from build123d import *

# Parameters (mm, degrees)
MAIN_LID_SKETCH_W   = 76.2
MAIN_LID_SKETCH_H   = 53.975
MAIN_LID_DEPTH      = 2.54
HOLE_CUT_DEPTH      = 47.758814744
HOLE_CUT_DEPTH_BACK = 47.758814744
HOLE_CUT_SKETCH_R   = 3.175
CORNER_FILLET_R     = 6.35


with BuildPart() as part:
    # Main Lid Sketch → Main Lid (new body)
    with BuildSketch(Plane(origin=(0, 0, 0), x_dir=(1, 0, 0), z_dir=(0, 1, 0))):
        Rectangle(MAIN_LID_SKETCH_W, MAIN_LID_SKETCH_H)
    extrude(amount=MAIN_LID_DEPTH)

    # Hole Cut Sketch → Hole Cut (cut, two sides: drawn at the far end of the back side and taken through both)
    with BuildSketch(Plane(origin=(0, 2.54, 0), x_dir=(1, 0, 0), z_dir=(0, 1, 0)).offset(-HOLE_CUT_DEPTH_BACK)):
        with Locations(Location((31.75, -20.6375, 0), (0, 0, 270))):
            Circle(HOLE_CUT_SKETCH_R)
        with Locations(Location((22.225, -20.6375, 0), (0, 0, 270))):
            Circle(HOLE_CUT_SKETCH_R)
        with Locations(Location((-31.75, -20.6375, 0), (0, 0, 270))):
            Circle(HOLE_CUT_SKETCH_R)
        with Locations(Location((-31.75, 20.6375, 0), (0, 0, 270))):
            Circle(HOLE_CUT_SKETCH_R)
        with Locations(Location((22.225, 20.6375, 0), (0, 0, 270))):
            Circle(HOLE_CUT_SKETCH_R)
        with Locations(Location((31.75, 20.6375, 0), (0, 0, 270))):
            Circle(HOLE_CUT_SKETCH_R)
    extrude(amount=HOLE_CUT_DEPTH + HOLE_CUT_DEPTH_BACK, mode=Mode.SUBTRACT)

    # Corner Fillet
    corner_fillet_edges = [part.edges().sort_by_distance(p)[0] for p in [
        (-38.1, 1.27, -26.9875),
        (38.1, 1.27, -26.9875),
        (38.1, 1.27, 26.9875),
        (-38.1, 1.27, 26.9875),
    ]]
    fillet(corner_fillet_edges, radius=CORNER_FILLET_R)


solid = part.part
Read the model definition and answer for the solid it produces. Units are mm, in the model's axes. Coordinates: 2 decimals unless noted, no trailing zeros. Loops run counter-clockwise (first coordinate to the right, second up) from the corner with the lowest first, then second, coordinate; pieces in that order, holes last. Notation, with made-up numbers: (77.5, -19.5) -> (102.5, -19.5) arc R22 cw to (102.5, 7.5) -> close; hole circle Ø6 at (39, 24.25). An arc over 180 degrees is marked (long way). Write item = value, one per line. Start each with the question number.
1) The part is cut by section B-B, the plane y = 2. State how many separate pieces and enclosed holes the cut face has, plus the area to 3 significant figures.
2) The part is cut by section A-A, the plane x = 31. Determine the outline of the cut face in (y, z).
3) The mould has two halves that part along Z. Classify faces 1 (the face through (36.19, 1.288, -25.177)), 2 (the face through (-36.29, 1.29, 25.08)), 3 (the face through (29.82, 1.25, -23.16)): pulls with the +Z half, pulls with the -Z half, needs draft (parallel to the pull), parting line crosses it, or undercut.
4) Find the intervals of material crossed by L1, parallel to Z at x = -31.75, y = 1.1; L2, parallel to X at y = 0.55, z = -21.5; L3, parallel to X at y = 0.15, z = 19, in increasing order. Write a range as from..to.
Result:
q1.separate_pieces = 1
q1.enclosed_holes = 6
q1.area = 3,890 mm²
q2.outline = (0, -26.99) -> (2.54, -26.99) -> (2.54, -23.72) -> (0, -23.72) -> close; (0, -17.55) -> (2.54, -17.55) -> (2.54, 17.55) -> (0, 17.55) -> close; (0, 23.72) -> (2.54, 23.72) -> (2.54, 26.99) -> (0, 26.99) -> close
q3.face_1 = pulls with the -Z half
q3.face_2 = pulls with the +Z half
q3.face_3 = undercut
q4.L1 = -26.99..-23.81, -17.46..17.46, 23.81..26.99
q4.L2 = -38.04..-34.81, -28.69..19.17, 25.28..28.69, 34.81..38.04
q4.L3 = -38.1..-34.47, -29.03..19.5, 24.95..29.03, 34.47..38.1
